Check sheet for the modelled part. Datum: model origin and axes. Units: mm. A direction names the side the tool comes from. Coordinates: 2 decimals unless noted, no trailing zeros. Write each loop counter-clockwise with the first axis right and the second up, starting at its lowest first coordinate (ties: lowest second). Pieces come first, ordered by that corner, then holes. Notation, with made-up numbers: (18.5, 4) - (68.5, 4) arc R13 cw to (68.5, 21) - close; hole circle Ø2 at (41.5, 79.25). An arc over 180 degrees is marked (long way). Use one line per item in the form item = value. Start each with the question number.
1. Scan lines: line 1 along X through (y, z) = (-5.75, -429.5); line 2 along X through (y, z) = (-1.25, -471); line 3 along Z through (x, y) = (175, -0.75). Record each from-to range of solid material in increasing order.
2. Draft check along X on faces 1 (the face through (0, -6, -273)), 2 (the face through (254.22, -5.916, -356.995)), 3 (the face through (207, -12, -265)), 4 (the face through (166.22, -5.916, -356.995)). Enter one of: +X half, -X half, draft (parallel to the pull), parting line (faces both ways), or undercut.
3. Cross-section at D-D on x = 167.5. Record the boundary of the cut face in (y, z).
4. Cross-section at A-A on y = -9.75. Record the boundary of the cut face in (x, z), then the cut area to 3 significant figures.
5. Cross-section at B-B on x = 342. Record the boundary of the cut face in (y, z), then the cut area to 3 significant figures.
6. Tool access check on faces 5 (the face through (342.22, -5.916, -356.995)), 6 (the face through (207, -6, 0)). Record the directions out of +Z, -Z, +X, -X, +Y, -Y that give a thin tool (end or side, any length) a straight path to the whole face; none if there is none.
7. Cross-section at C-C on z = -375.5. Record the boundary of the cut face in (x, y), then the cut area to 3 significant figures.
8. Go/stop test with a flat-tipped pin: pin 1 Ø12 at (x, z) = (344, -400.5) entering from +Y. Record where the tip stops, or that it passes through.
```python
from build123d import *

# Parameters (mm, degrees)
SKETCH_W  = 420
SKETCH_H  = 538
PAD_DEPTH = 12


with BuildPart() as part:
    # Sketch → Pad (new body)
    with BuildSketch(Plane.XZ):
        with Locations((210, -269)):
            Rectangle(SKETCH_W, SKETCH_H)
        with BuildLine():
            ThreePointArc((88, -366.992235), (78, -356.992235), (68, -366.992235))
            Line((68, -366.992235), (68, -468))
            ThreePointArc((68, -468), (78, -478), (88, -468))
            Line((88, -366.992235), (88, -468))
        make_face(mode=Mode.SUBTRACT)
        with BuildLine():
            ThreePointArc((264, -366.992235), (254, -356.992235), (244, -366.992235))
            Line((244, -366.992235), (244, -468))
            ThreePointArc((244, -468), (254, -478), (264, -468))
            Line((264, -366.992235), (264, -468))
        make_face(mode=Mode.SUBTRACT)
        with BuildLine():
            ThreePointArc((352, -366.992235), (342, -356.992235), (332, -366.992235))
            Line((332, -366.992235), (332, -468))
            ThreePointArc((332, -468), (342, -478), (352, -468))
            Line((352, -366.992235), (352, -468))
        make_face(mode=Mode.SUBTRACT)
        with BuildLine():
            ThreePointArc((176, -366.992235), (166, -356.992235), (156, -366.992235))
            Line((156, -366.992235), (156, -468))
            ThreePointArc((156, -468), (166, -478), (176, -468))
            Line((176, -366.992235), (176, -468))
        make_face(mode=Mode.SUBTRACT)
    extrude(amount=PAD_DEPTH)


solid = part.part
```
Final values:
q1.line_1 = 0 to 68, 88 to 156, 176 to 244, 264 to 332, 352 to 420
q1.line_2 = 0 to 68.46, 87.54 to 156.46, 175.54 to 244.46, 263.54 to 332.46, 351.54 to 420
q1.line_3 = -538 to -472.36, -362.63 to 0
q2.face_1 = -X half
q2.face_2 = undercut
q2.face_3 = draft
q2.face_4 = undercut
q3.outline = (-12, -538) - (0, -538) - (0, -477.89) - (-12, -477.89) - close; (-12, -357.11) - (0, -357.11) - (0, 0) - (-12, 0) - close
q4.outline = (0, -538) - (420, -538) - (420, 0) - (0, 0) - close; hole (68, -468) arc R10 ccw to (88, -468) - (88, -366.99) arc R10 ccw to (68, -366.99) - close; hole (156, -468) arc R10 ccw to (176, -468) - (176, -366.99) arc R10 ccw to (156, -366.99) - close; hole (244, -468) arc R10 ccw to (264, -468) - (264, -366.99) arc R10 ccw to (244, -366.99) - close; hole (332, -468) arc R10 ccw to (352, -468) - (352, -366.99) arc R10 ccw to (332, -366.99) - close
q4.area = 217,000 mm²
q5.outline = (-12, -538) - (0, -538) - (0, -478) - (-12, -478) - close; (-12, -356.99) - (0, -356.99) - (0, 0) - (-12, 0) - close
q5.area = 5,000 mm²
q6.face_5 = +Y, -Y
q6.face_6 = +Z, +X, -X, +Y, -Y
q7.outline = (0, -12) - (68, -12) - (68, 0) - (0, 0) - close; (88, -12) - (156, -12) - (156, 0) - (88, 0) - close; (176, -12) - (244, -12) - (244, 0) - (176, 0) - close; (264, -12) - (332, -12) - (332, 0) - (264, 0) - close; (352, -12) - (420, -12) - (420, 0) - (352, 0) - close
q7.area = 4,080 mm²
q8.pin_1 = through
